Verification items for the finished model (mm, model axes). Coordinates: 2 decimals unless noted, no trailing zeros. Order: outer loops, then holes, each group sorted by start corner. A loop starts at its lowest first (then second) coordinate and runs counter-clockwise, first axis right, second up. Notation, with made-up numbers: M 45.25,64.25 L 59.25,64.25 A32 ccw 59.25,103.25 Z; hole C 85,29.25 d10. An arc over 180 degrees is marked long. Return JSON: item names as keys, results as strings. Group by question number.
1. Section check B-B, the plane y = 1.75. Record the cut outline in (x, z).
2. Section check D-D, the plane y = 5. Record the cut outline in (x, z).
3. Material ranges on line 1 along Y through (x, z) = (-3, 3.5); line 2 along X through (y, z) = (-6, 0.5); line 3 along X through (y, z) = (-3.25, 2.25), recorded low to high.
4. Gauge pin test, flat ends, axial feed: pin 1 (1 mm diameter, centred on x = 3.5, y = 1.5, fed in from -Z); pin 2 (4 mm diameter, centred on x = 6, z = 1, fed in from +Y); pin 3 (1.5 mm diameter, centred on x = 6, z = 1.5, fed in from +Y); pin 4 (6 mm diameter, centred on x = 3, y = 2, fed in from -Z). Record the tip position at first contact, or that the pin passes through.
5. Section check A-A, the plane x = 3. Record the cut outline in (y, z), plus the area to 3 significant figures.
6. Mould release check, pull along X, two halves, no side actions. Record for faces 1 (the cylindrical face through (4.9, -3.8, 3.5)), 2 (the flat face through (4.27, 6.23, 3.45)), 3 (the flat face through (-4, -6, 0)), 4 (the flat face through (-4.39, -8.77, 3.45)): +X half, -X half, draft (parallel to the pull), parting line (faces both ways), or undercut.
7. Section check C-C, the plane z = 1. Record the cut outline in (x, y).
Autodesk Inventor part; units mm, degrees
ref_plane "YZ Plane" through (0, 0, 0) normal (1, 0, 0) x (0, 1, 0)
ref_plane "XZ Plane" through (0, 0, 0) normal (0, 1, 0) x (-1, 0, 0)
ref_plane "XY Plane" through (0, 0, 0) normal (0, 0, 1) x (1, 0, 0)
sketch "Sketch1" plane through (0, 0, 0) normal (0, 0, 1) x (1, 0, 0)
  line L0 (0, 12.846) -> (0, -12.1789)
  line L1 (0, 8.6963) -> (-8.6603, 3.6963)
  line L2 (-8.6603, 3.6963) -> (-8.6603, -6.3037)
  line L3 (-8.6603, -6.3037) -> (0, -11.3037)
  line L4 (0, 8.6963) -> (8.6603, 3.6963)
  line L5 (8.6603, 3.6963) -> (8.6603, -6.3037)
  line L6 (8.6603, -6.3037) -> (0, -11.3037)
  point P0 (0, 0)
  dimension "d0" = 120
  dimension "d1" = 120
  dimension "d2" = 10
  dimension "d4" = 5
  dimension "d16" = 9.7893
  dimension "d17" = 20.9142
  dimension "d18" = 0.758
extrude "Extrusion1" add sketch "Sketch1" along normal blind 7
sketch "Sketch2" plane through (0, 0, 7) normal (0, 0, 1) x (1, 0, 0)
  line L0 (0, 10.2692) -> (0, -14.045)
  line L1 (8.6603, -6.3037) -> (8.6603, 3.6963)
  line L2 (8.6603, -1.3037) -> (-8.6603, -1.3037)
  line L3 (-8.6603, 3.6963) -> (-8.6603, -6.3037)
  point P0 (0, 0)
  point P1 (0, -1.3037)
  dimension "d22" = 8.6602
  dimension "d23" = 23.1456
  dimension "d24" = 25.4826
hole "Hole1" at (0, -1.3037, 7) direction (0, 0, -1) diameter 11 end through all
thread "Thread2"
equation "\"d4\" = 0.5 * d2"
properties part number "mutter"
Answers follow:
{
 "1": {"outline": "M -8.66,0 L -4.57,0 L -4.57,7 L -8.66,7 Z; M 4.57,0 L 8.66,0 L 8.66,7 L 4.57,7 Z"},
 "2": {"outline": "M -6.4,0 L 6.4,0 L 6.4,7 L -6.4,7 Z"},
 "3": {"line 1": "-9.57 to -5.91, 3.31 to 6.96", "line 2": "-8.66 to -2.86, 2.86 to 8.66", "line 3": "-8.66 to -5.14, 5.14 to 8.66"},
 "4": {"pin 1": "through", "pin 2": "y = 6.39", "pin 3": "y = 5.67", "pin 4": "z = 0"},
 "5": {"outline": "M -9.57,0 L -5.91,0 L -5.91,7 L -9.57,7 Z; M 3.31,0 L 6.96,0 L 6.96,7 L 3.31,7 Z", "area": "51.2 mm^2"},
 "6": {"face 1": "undercut", "face 2": "+X half", "face 3": "draft", "face 4": "-X half"},
 "7": {"outline": "M -8.66,-6.3 L 0,-11.3 L 8.66,-6.3 L 8.66,3.7 L 0,8.7 L -8.66,3.7 Z; hole C 0,-1.3 d11"}
}
